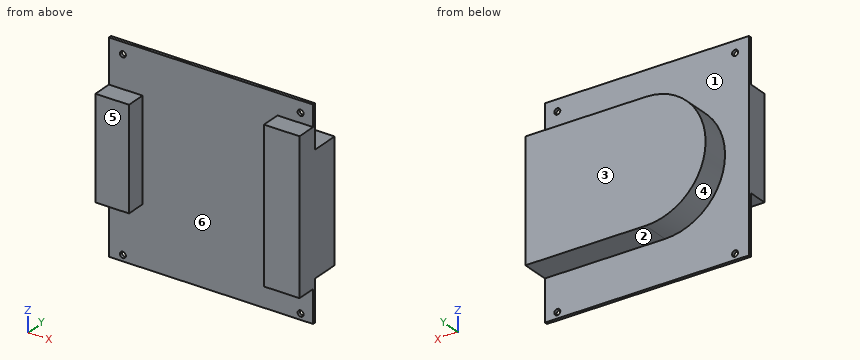
```python
from build123d import *

# Parameters (mm, degrees)
SKETCH1_W           = 104.14
SKETCH1_H           = 104.14
SKETCH1_R           = 1.524
BOSS_EXTRUDE1_DEPTH = 1.524
BOSS_EXTRUDE2_DEPTH = 14.224
SKETCH3_W           = 18.136210303
SKETCH3_H           = 76.873137305
BOSS_EXTRUDE3_DEPTH = 9.906
SKETCH5_W           = 17.139817269
SKETCH5_H           = 51.595631098
BOSS_EXTRUDE4_DEPTH = 9.906


with BuildPart() as part:
    # Sketch1 → Boss-Extrude1 (new body)
    with BuildSketch(Plane(origin=(0, 0, 0), x_dir=(1, 0, 0), z_dir=(0, 1, 0))):
        with Locations((52.07, 52.07)):
            Rectangle(SKETCH1_W, SKETCH1_H)
        with Locations((7.112, 101.092)):
            Circle(SKETCH1_R, mode=Mode.SUBTRACT)
        with Locations((97.79, 101.092)):
            Circle(SKETCH1_R, mode=Mode.SUBTRACT)
        with Locations((7.112, 5.842)):
            Circle(SKETCH1_R, mode=Mode.SUBTRACT)
        with Locations((97.79, 5.842)):
            Circle(SKETCH1_R, mode=Mode.SUBTRACT)
    extrude(amount=BOSS_EXTRUDE1_DEPTH)

    # Sketch2 → Boss-Extrude2 (add)
    with BuildSketch(Plane(origin=(0, 1.524, 0), x_dir=(1, 0, 0), z_dir=(0, 1, 0))):
        with BuildLine():
            Line((104.14, 22.024034198), (104.14, 83.197819697))
            Line((104.14, 83.197819697), (42.798644119, 83.197819697))
            ThreePointArc((42.798644119, 83.197819697), (64.426843398, 74.239126226), (73.385536869, 52.610926948))
            ThreePointArc((73.385536869, 52.610926948), (64.426843398, 30.982727669), (42.798644119, 22.024034198))
            Line((42.798644119, 22.024034198), (104.14, 22.024034198))
        make_face()
        with BuildLine():
            ThreePointArc((73.385536869, 52.610926948), (64.426843398, 74.239126226), (42.798644119, 83.197819697))
            Line((42.798644119, 83.197819697), (42.798644119, 22.024034198))
            ThreePointArc((42.798644119, 22.024034198), (64.426843398, 30.982727669), (73.385536869, 52.610926948))
        make_face()
        with BuildLine():
            Line((42.798644119, 22.024034198), (42.798644119, 83.197819697))
            ThreePointArc((42.798644119, 83.197819697), (12.211751369, 52.610926948), (42.798644119, 22.024034198))
        make_face()
    extrude(amount=BOSS_EXTRUDE2_DEPTH)

    # Sketch3 → Boss-Extrude3 (add)
    with BuildSketch(Plane.XZ):
        with Locations((95.071894848, -49.113594912)):
            Rectangle(SKETCH3_W, SKETCH3_H)
    extrude(amount=BOSS_EXTRUDE3_DEPTH)

    # Sketch5 → Boss-Extrude4 (add)
    with BuildSketch(Plane.XZ):
        with Locations((8.569908635, -48.177785321)):
            Rectangle(SKETCH5_W, SKETCH5_H)
    extrude(amount=BOSS_EXTRUDE4_DEPTH)


solid = part.part
```
Geometry: final body of the model. Coordinates: model frame, mm. Face numbers are marked on the shaded views. A direction names the side the tool comes from. Round coordinates to 2 decimals unless told otherwise and drop trailing zeros. Write each loop counter-clockwise with the first axis right and the second up, starting at its lowest first coordinate (ties: lowest second). Pieces come first, ordered by that corner, then holes. Notation, with made-up numbers: (24.25, 65) -> (29.25, 65) arc R28 ccw to (29.25, 100) -> close; hole circle Ø10 at (28.5, -37). An arc over 180 degrees is marked (long way). Use CSV: the item, a comma, the result in double quotes. Start each with the question number.
Q1. Section C-C (x = 63). Return loops of the section in (y, z).
Q2. First-contact query: pin 1 Ø4 at (x, z) = (7.112, -101.092) entering from -Y; pin 2 Ø8 at (x, y) = (9, -5.5) entering from +Z; pin 3 Ø2.5 at (x, z) = (7.112, -5.842) entering from -Y; pin 4 Ø8 at (x, y) = (12.5, -5.5) entering from -Z. Flat tips, straight axial feed; report the tip coordinate or a pass-through.
Q3. Section D-D (y = 5). Return loops of the section in (x, z).
Q4. Pull-direction query (X, two-part tool) for the marked faces 4, 5 and 6; classes: pulls with the +X half, pulls with the -X half, needs draft (parallel to the pull), parting line crosses it, or undercut.
Q5. Reachability of the marked faces 1, 2 and 3 from +Z, -Z, +X, -X, +Y, -Y: full face, straight path, thin tool, end or side. Return the list, or none.
Q6. Section B-B (z = -12.5). Return loops of the section in (x, y), plus the area to 3 significant figures.
Q7. Line query: L1, parallel to Z at x = 97.79, y = 1.1; L2, parallel to X at y = -7.75, z = -32; L3, parallel to Y at x = 45.5, z = -96.5. Output: solid intervals per line, ascending.
Q8. Section A-A (x = 97.79). Return loops of the section in (y, z), plus the area to 3 significant figures.
Result sheet:
1,outline,"(0, -104.14) -> (1.52, -104.14) -> (1.52, -83.2) -> (15.75, -83.2) -> (15.75, -22.02) -> (1.52, -22.02) -> (1.52, 0) -> (0, 0) -> close"
2,pin 1,"y = 0"
2,pin 2,"z = -22.38"
2,pin 3,"through"
2,pin 4,"z = -73.98"
3,outline,"(42.8, -83.2) -> (104.14, -83.2) -> (104.14, -22.02) -> (42.8, -22.02) arc R30.59 ccw to start"
4,face 4,"pulls with the -X half"
4,face 5,"needs draft"
4,face 6,"undercut"
5,face 1,"-X, +Y"
5,face 2,"-Z, +X, -X, +Y"
5,face 3,"+Z, -Z, +X, -X, +Y"
6,outline,"(0, 0) -> (86, 0) -> (86, -9.91) -> (104.14, -9.91) -> (104.14, 1.52) -> (0, 1.52) -> close"
6,area,"338 mm²"
7,L1,"-104.14 to -102.62, -99.57 to -7.37, -4.32 to 0"
7,L2,"0 to 17.14, 86 to 104.14"
7,L3,"0 to 1.52"
8,outline,"(-9.91, -87.55) -> (0, -87.55) -> (0, -99.57) -> (1.52, -99.57) -> (1.52, -83.2) -> (15.75, -83.2) -> (15.75, -22.02) -> (1.52, -22.02) -> (1.52, -7.37) -> (0, -7.37) -> (0, -10.68) -> (-9.91, -10.68) -> close; (0, -104.14) -> (1.52, -104.14) -> (1.52, -102.62) -> (0, -102.62) -> close; (0, -4.32) -> (1.52, -4.32) -> (1.52, 0) -> (0, 0) -> close"
8,area,"1,780 mm²"
